Part model, mm, in its own coordinate system. A direction names the side the tool comes from. Round coordinates to 2 decimals unless told otherwise and drop trailing zeros. Write each loop counter-clockwise with the first axis right and the second up, starting at its lowest first coordinate (ties: lowest second). Pieces come first, ordered by that corner, then holes. Notation, with made-up numbers: M 5.5,33 L 42.5,33 A16 cw 42.5,64 Z; hole C 27.5,70.25 d10. An arc over 180 degrees is marked long. Use a Markdown table: item, result. Add a question column.
1) Drop flat-ended pins along their axis: P1, Ø3, axis at x = 1.5, z = 11.5, coming from the +Y side (3 decimals); P2, Ø3, axis at x = 5, y = -13, coming from the +Z side; P3, Ø2.5, axis at y = 3.5, z = -6.5, coming from the +X side (3 decimals). Give the stop position or say it passes through.
2) Slice it at A-A on y = -3.81. Write the cut outline in (x, z) (3 decimals).
3) Wall check: probe 1 along Y at (x, z) = (-4.25, 21.5) (3 decimals); probe 2 along X at (y, z) = (6.25, -10) (3 decimals); probe 3 along X at (y, z) = (-6, -11.5) (3 decimals). Give the ranges that are in metal, low to high.
4) Slice it at C-C on z = 1.5. Write the cut outline in (x, y) (3 decimals), plus the area to 3 significant figures.
5) Two-plate mould, pull along Z, no slides. Class faces 6 (the face through (-3.6, -13.9, 22.555)), 7 (the face through (-3.264, -3.771, -23.113)), 8 (the face through (0, -15.875, -19)): released by +Z, released by -Z, zero draft, split by the parting line, or undercut.
6) Slice it at D-D on x = -5.5. Write the cut outline in (y, z) (3 decimals).
7) Slice it at B-B on y = 2. Write the cut outline in (x, z) (3 decimals), plus the area to 3 significant figures.
8) Which spindle directions (+Z, -Z, +X, -X, +Y, -Y) get a long thin tool onto all of the face, cutting with end or side? Do faces 1 (the face through (-3.175, 3, 0)), 2 (the face through (6.95, -4.89, -21.66)), 3 (the face through (-3.269, -10.357, 23.998)), 4 (the face through (8.255, -6, -22)), 5 (the face through (7, 0, -19.05)). Say none if no direction does.
```python
from build123d import *

# Parameters (mm, degrees)
SKETCH2_W                                      = 19.05
SKETCH2_H                                      = 19.05
BOSS_EXTRUDE1_DEPTH                            = 25.4
CUT_EXTRUDE1_DEPTH                             = 54.497649479
SKETCH6_W                                      = 1.27
SKETCH6_H                                      = 11.43
SKETCH6_H_2                                    = 1.27
SKETCH6_W_2                                    = 3.81
CUT_EXTRUDE2_DEPTH                             = 54.497649479
CUT_EXTRUDE3_REACH                             = 35.148
SKETCH7_W                                      = 38.1
SKETCH7_H                                      = 13.97
SKETCH8_W                                      = 19.05
SKETCH8_H                                      = 6.35
BOSS_EXTRUDE2_DEPTH                            = 12.7
CBORE_FOR_4_SOCKET_HEAD_CAP_SCREW1_D           = 2.9464
CBORE_FOR_4_SOCKET_HEAD_CAP_SCREW1_DEPTH       = 12.7
CBORE_FOR_4_SOCKET_HEAD_CAP_SCREW1_CBORE_D     = 5.55752
CBORE_FOR_4_SOCKET_HEAD_CAP_SCREW1_CBORE_DEPTH = 2.8448
F_2_CLEARANCE_HOLE1_D                          = 2.4384
F_2_CLEARANCE_HOLE1_DEPTH                      = 5.08
F_2_56_TAPPED_HOLE1_D                          = 1.778


with BuildPart() as part:
    # Sketch2 → Boss-Extrude1 (new, symmetric)
    with BuildSketch(Plane.XY):
        Rectangle(SKETCH2_W, SKETCH2_H)
    extrude(amount=BOSS_EXTRUDE1_DEPTH, both=True)

    # Sketch4 → Cut-Extrude1 (cut, through all)
    with BuildSketch(Plane(origin=(-1.506852909, 3.110534069, 25.4), x_dir=(1, 0, 0), z_dir=(0, 0, 1))):
        Polygon((-8.018147091, 6.414465931), (-8.018147091, 3.874465931), (-1.668147091, 3.874465931), (-1.668147091, -3.745534069), (4.681852909, -3.745534069), (4.681852909, 3.874465931), (11.031852909, 3.874465931), (11.031852909, 6.414465931), align=None)
    extrude(amount=-CUT_EXTRUDE1_DEPTH, mode=Mode.SUBTRACT)

    # Sketch6 → Cut-Extrude2 (cut, through all)
    with BuildSketch(Plane(origin=(-1.506852909, 3.110534069, 25.4), x_dir=(1, 0, 0), z_dir=(0, 0, 1))):
        with Locations((5.316852909, -3.110534069)):
            Rectangle(SKETCH6_W, SKETCH6_H)
        with Locations((5.316852909, -9.460534069)):
            Rectangle(SKETCH6_W, SKETCH6_H_2)
        with Locations((7.856852909, -9.460534069)):
            Rectangle(SKETCH6_W_2, SKETCH6_H_2)
    extrude(amount=-CUT_EXTRUDE2_DEPTH, mode=Mode.SUBTRACT)

    # Cut-Extrude3: up to this face of the body (flat: up to its plane)
    cut_extrude3_end = Plane(part.part.faces().sort_by_distance((3.175, 6.35, 0))[0])
    # Sketch7 → Cut-Extrude3 (cut, up to the picked face)
    with BuildSketch(Plane(origin=(9.525, 0, 0), x_dir=(0, 0, -1), z_dir=(1, 0, 0)), mode=Mode.PRIVATE) as cut_extrude3_sk1:
        Rectangle(SKETCH7_W, SKETCH7_H)
    cut_extrude3_tool1 = split(extrude(cut_extrude3_sk1.sketch, amount=-CUT_EXTRUDE3_REACH, mode=Mode.PRIVATE), bisect_by=cut_extrude3_end, keep=Keep.BOTH, mode=Mode.PRIVATE)
    add(cut_extrude3_tool1.solids().sort_by(Axis((9.525, 0, 0), (-1, 0, 0)))[0], mode=Mode.SUBTRACT)

    # Sketch8 → Boss-Extrude2 (add)
    with BuildSketch(Plane.XY.offset(25.4)):
        with Locations((0, -12.7)):
            Rectangle(SKETCH8_W, SKETCH8_H)
    boss_extrude2 = extrude(amount=-BOSS_EXTRUDE2_DEPTH)

    # Mirror1: Boss-Extrude2 across plane
    add(boss_extrude2.mirror(Plane.XY))

    # CBORE for #4 Socket Head Cap Screw1
    with Locations(Plane.XY.offset(25.4)):
        with Locations((-4.7625, -12.7), (4.7625, -12.7)):
            CounterBoreHole(CBORE_FOR_4_SOCKET_HEAD_CAP_SCREW1_D / 2, CBORE_FOR_4_SOCKET_HEAD_CAP_SCREW1_CBORE_D / 2, CBORE_FOR_4_SOCKET_HEAD_CAP_SCREW1_CBORE_DEPTH, depth=CBORE_FOR_4_SOCKET_HEAD_CAP_SCREW1_DEPTH)

    # #2 Clearance Hole1
    with Locations(Plane(origin=(9.525, 0, 0), x_dir=(0, 0, -1), z_dir=(1, 0, 0))):
        with Locations((-22.225, -3.81), (22.225, -3.81)):
            Hole(F_2_CLEARANCE_HOLE1_D / 2, depth=F_2_CLEARANCE_HOLE1_DEPTH)

    # #2-56 Tapped Hole1 (through all)
    with Locations(Plane(origin=(3.175, 0, 0), x_dir=(0, 0, -1), z_dir=(1, 0, 0))):
        with Locations((-22.225, -3.81), (22.225, -3.81)):
            Hole(F_2_56_TAPPED_HOLE1_D / 2)


solid = part.part
```
Entries:
| question | item | result |
|---|---|---|
| 1 | P1 | stops at y = -0.635 |
| 1 | P2 | stops at z = 22.56 |
| 1 | P3 | stops at x = -3.175 |
| 2 | outline | M -9.525,-25.4 L 3.175,-25.4 L 3.175,-23.114 L -9.525,-23.114 Z; M -9.525,-21.336 L 3.175,-21.336 L 3.175,21.336 L -9.525,21.336 Z; M -9.525,23.114 L 3.175,23.114 L 3.175,25.4 L -9.525,25.4 Z; M 4.445,-25.4 L 9.525,-25.4 L 9.525,-23.444 L 4.445,-23.444 Z; M 4.445,-21.006 L 9.525,-21.006 L 9.525,-19.05 L 4.445,-19.05 Z; M 4.445,19.05 L 9.525,19.05 L 9.525,21.006 L 4.445,21.006 Z; M 4.445,23.444 L 9.525,23.444 L 9.525,25.4 L 4.445,25.4 Z |
| 3 | probe 1 | y = -15.875 to -14.081, -11.319 to -4.324, -3.296 to 6.985 |
| 3 | probe 2 | x = -9.525 to -3.175 |
| 3 | probe 3 | x = -9.525 to 3.175 |
| 4 | outline | M -9.525,-9.525 L 9.525,-9.525 L 9.525,-6.985 L 3.175,-6.985 L 3.175,-0.635 L -3.175,-0.635 L -3.175,6.985 L -9.525,6.985 Z |
| 4 | area | 177 mm^2 |
| 5 | face 6 | released by +Z |
| 5 | face 7 | undercut |
| 5 | face 8 | zero draft |
| 6 | outline | M -15.875,-25.4 L 6.985,-25.4 L 6.985,25.4 L -10.021,25.4 L -10.021,22.555 L -11.425,22.555 L -11.425,12.7 L -9.525,12.7 L -9.525,-12.7 L -15.875,-12.7 Z; M -15.875,12.7 L -13.975,12.7 L -13.975,22.555 L -15.379,22.555 L -15.379,25.4 L -15.875,25.4 Z; hole C -3.81,-22.225 d1.778; hole C -3.81,22.225 d1.778 |
| 7 | outline | M -9.525,-25.4 L -3.175,-25.4 L -3.175,25.4 L -9.525,25.4 Z; M 4.445,-25.4 L 9.525,-25.4 L 9.525,-19.05 L 4.445,-19.05 Z; M 4.445,19.05 L 9.525,19.05 L 9.525,25.4 L 4.445,25.4 Z |
| 7 | area | 387 mm^2 |
| 8 | face 1 | +Z, -Z, +Y |
| 8 | face 2 | +X |
| 8 | face 3 | +Z |
| 8 | face 4 | +Z, -Z |
| 8 | face 5 | +X, +Y |
